Can you work these out from the model? Positions are in its coordinate system, mm. A direction names the side the tool comes from. Round coordinates to 2 decimals unless told otherwise and drop trailing zeros. Write each loop counter-clockwise with the first axis right and the second up, starting at its lowest first coordinate (ties: lowest second). Pieces come first, ordered by that corner, then holes. Notation, with made-up numbers: M -14,-23 L 3,-23 A33 cw 3,9 Z; hole C 37.25,-40 d2. An arc over 180 degrees is marked long. Answer as a JSON object with one key per item and string values. Group by question number.
1) Suppose I cut it at B-B, the plane y = -65. Write out the boundary of the cut face in (x, z).
2) Please list where these lines run through material, in increasing order: L1, parallel to Y at x = 217, z = -6.25; L2, parallel to Y at x = 101, z = -9; L3, parallel to X at y = -85, z = -5.25. Write a range as [from, to].
3) Suppose I cut it at C-C, the plane x = 193. Write out the boundary of the cut face in (y, z).
4) I'm going to push flat-ended pins straight in: pin 1 Ø2 at (y, z) = (-81.5, -2) entering from +X; pin 2 Ø6 at (y, z) = (-106.5, -1.5) entering from +X; pin 3 Ø4 at (x, z) = (107.5, -8.5) entering from -Y. Where does each tip first touch, or does it pass through?
5) If we mould it in two halves opening along Z, with no side actions, what happens to faces 5 (the flat face through (130, -39, -10)), 6 (the flat face through (262, -115, -7.5)), 7 (the flat face through (-8, -10, -5))? For each: +Z half, -Z half, draft (parallel to the pull), parting line (faces both ways), or undercut.
6) On a 3-axis mill with a long thin cutter (end or side, diameter ignored), from which of +Z, -Z, +X, -X, +Y, -Y can I reach the whole of each face in a straight line? I mean faces 1 (the flat face through (-4, -8, -1.2)), 2 (the flat face through (259.122, -112.334, -5.035)), 3 (the flat face through (-4, -19.5, -5)), 4 (the flat face through (258.8, -117.75, -4.96)). Say none if no direction works.
7) Suppose I cut it at A-A, the plane z = -6. Write out the boundary of the cut face in (x, y), and give its area (3 significant figures).
Autodesk Inventor part; units mm, degrees
ref_plane "YZ Plane" through (0, 0, 0) normal (1, 0, 0) x (0, 1, 0)
ref_plane "XZ Plane" through (0, 0, 0) normal (0, 1, 0) x (-1, 0, 0)
ref_plane "XY Plane" through (0, 0, 0) normal (0, 0, 1) x (1, 0, 0)
sketch "Sketch1" plane through (0, 0, 0) normal (0, 0, 1) x (1, 0, 0)
  arc A0 (381.5, -381.5) -> (0, 0) centre (0, -381.5) ccw
  line L0 (-227, 0) -> (0, 0)
  line L1 (381.5, -381.5) -> (381.5, -681.5)
  line L2 (-227, -19.5) -> (0, -19.5)
  arc A1 (362, -381.5) -> (0, -19.5) centre (0, -381.5) ccw
  line L3 (362, -381.5) -> (362, -681.5)
  line L4 (-8, 0) -> (-8, -19.5)
  line L5 (381.5, -389.5) -> (362, -389.5)
  line L6 (269.7612, -111.7388) -> (255.9727, -125.5273)
  dimension "d0" = 19.5
  dimension "d1" = 8
  dimension "d2" = 8
extrude "Extrusion1" add sketch "Sketch1" against normal blind 10 contours L6 A1 L2 L4 L0 A0
sketch "Sketch2" plane through (-8, -19.5, 0) normal (-1, 0, 0) x (0, 0, 1)
  line L0 (0, 19.5) -> (0, 0)
  line L1 (0, 19.5) -> (-10, 19.5)
  line L2 (-10, 0) -> (-10, 19.5)
  line L3 (0, 0) -> (-10, 0)
  line L4 (-1.2, 14.5) -> (-4.2, 14.5)
  line L5 (-4.2, 14.5) -> (-4.2, 9.5)
  line L6 (-4.2, 9.5) -> (-1.2, 9.5)
  line L7 (-1.2, 9.5) -> (-1.2, 14.5)
  line L8 (-1.2, 14.5) -> (-4.2, 9.5) construction
  line L9 (-4.2, 14.5) -> (-1.2, 9.5) construction
  point P0 (0, 19.5)
  point P1 (-2.7, 12)
  dimension "d5" = 3
  dimension "d6" = 5
  dimension "d7" = 1.2
  dimension "d8" = 5
extrude "Extrusion2" cut sketch "Sketch2" against normal blind 7.1 contours L7 L6 L5 L4
sketch "Sketch3" plane through (255.9727, -125.5273, 0) normal (0.7071, -0.7071, 0) x (-0.7071, -0.7071, 0)
  line L0 (0, 0) -> (-19.5, 0)
  line L1 (0, 0) -> (0, 10)
  line L2 (-19.5, 10) -> (0, 10)
  line L3 (-19.5, 0) -> (-19.5, 10)
  line L4 (-15.5, 2.5) -> (-7.5, 2.5)
  line L5 (-7.5, 2.5) -> (-7.5, 7.5)
  line L6 (-7.5, 7.5) -> (-15.5, 7.5)
  line L7 (-15.5, 7.5) -> (-15.5, 2.5)
  line L8 (-15.5, 2.5) -> (-7.5, 7.5) construction
  line L9 (-7.5, 2.5) -> (-15.5, 7.5) construction
  line L10 (-15.7, 2.3) -> (-7.3, 2.3)
  line L11 (-7.3, 2.3) -> (-7.3, 7.7)
  line L12 (-7.3, 7.7) -> (-15.7, 7.7)
  line L13 (-15.7, 7.7) -> (-15.7, 2.3)
  point P0 (92.2388, 0)
  point P1 (-11.5, 5)
  point P2 (-15.5, 5)
  point P3 (-19.5, 5)
  dimension "d11" = 8
  dimension "d12" = 5
  dimension "d13" = 4
  dimension "d16" = 0.2
extrude "Extrusion3" cut sketch "Sketch3" against normal blind 7.1 contours L7 L6 L5 L4
properties part number "SEPARADOR_3"
Results:
{
 "1": {"outline": "M 175.7,-10 L 213,-10 L 213,0 L 175.7,0 Z"},
 "2": {"L1": "[-91.75, -67.73]", "L2": "[-33.88, -13.61]", "L3": "[207.68, 240.06]"},
 "3": {"outline": "M -75.24,-10 L -52.42,-10 L -52.42,0 L -75.24,0 Z"},
 "4": {"pin 1": "x = 236.94", "pin 2": "x = 267.5", "pin 3": "y = -36.46"},
 "5": {"face 5": "-Z half", "face 6": "undercut", "face 7": "draft"},
 "6": {"face 1": "-X", "face 2": "none", "face 3": "+Z, -Z, -X, -Y", "face 4": "+X"},
 "7": {"outline": "M -8,-19.5 L 0,-19.5 A362 cw 255.97,-125.53 L 261.28,-120.22 L 256.25,-115.2 L 261.91,-109.55 L 266.93,-114.57 L 269.76,-111.74 A381.5 ccw 0,0 L -8,0 Z", "area": "5,790 mm^2"}
}
